from build123d import *

# Parameters (mm, degrees)
ESQUISSE1_R             = 50
ESQUISSE1_R_2           = 4.25
BOSS_EXTRU_1_DEPTH      = 3
ESQUISSE2_R             = 4.25
BOSS_EXTRU_2_DEPTH      = 25
ENL_V_MAT_EXTRU_1_DEPTH = 20
CONG_1_R                = 2


with BuildPart() as part:
    # Esquisse1 → Boss.-Extru.1 (new body)
    with BuildSketch(Plane(origin=(0, 0, 0), x_dir=(1, 0, 0), z_dir=(0, 1, 0))):
        with Locations(Location((0, 0, 0), (0, 0, 270))):
            Circle(ESQUISSE1_R)
        with Locations(Location((0, 0, 0), (0, 0, 270))):
            Circle(ESQUISSE1_R_2, mode=Mode.SUBTRACT)
    extrude(amount=BOSS_EXTRU_1_DEPTH)

    # Esquisse2 → Boss.-Extru.2 (add)
    with BuildSketch(Plane(origin=(0, 3, 0), x_dir=(1, 0, 0), z_dir=(0, 1, 0))):
        with BuildLine():
            Line((9.886859967, 1.5), (47.476309882, 1.5))
            ThreePointArc((47.476309882, 1.5), (47.5, 0), (47.476309882, -1.5))
            Line((47.476309882, -1.5), (9.886859967, -1.5))
            ThreePointArc((9.886859967, -1.5), (7.071067812, -7.071067812), (1.5, -9.886859967))
            Line((1.5, -9.886859967), (1.5, -47.476309882))
            ThreePointArc((1.5, -47.476309882), (0, -47.5), (-1.5, -47.476309882))
            Line((-1.5, -47.476309882), (-1.5, -9.886859967))
            ThreePointArc((-1.5, -9.886859967), (-7.071067812, -7.071067812), (-9.886859967, -1.5))
            Line((-9.886859967, -1.5), (-47.476309882, -1.5))
            ThreePointArc((-47.476309882, -1.5), (-47.5, 0), (-47.476309882, 1.5))
            Line((-47.476309882, 1.5), (-9.886859967, 1.5))
            ThreePointArc((-9.886859967, 1.5), (-7.071067812, 7.071067812), (-1.5, 9.886859967))
            Line((-1.5, 9.886859967), (-1.5, 47.476309882))
            ThreePointArc((-1.5, 47.476309882), (0, 47.5), (1.5, 47.476309882))
            Line((1.5, 47.476309882), (1.5, 9.886859967))
            ThreePointArc((1.5, 9.886859967), (7.071067812, 7.071067812), (9.886859967, 1.5))
        make_face()
        with Locations(Location((0, 0, 0), (0, 0, 270))):
            Circle(ESQUISSE2_R, mode=Mode.SUBTRACT)
    extrude(amount=BOSS_EXTRU_2_DEPTH)

    # Esquisse3 → Enlèv. mat.-Extru.1 (cut)
    with BuildSketch(Plane(origin=(0, 28, 0), x_dir=(1, 0, 0), z_dir=(0, 1, 0))):
        Polygon((7.736493607, 0), (3.868246804, 6.7), (-3.868246804, 6.7), (-7.736493607, 0), (-3.868246804, -6.7), (3.868246804, -6.7), align=None)
    extrude(amount=-ENL_V_MAT_EXTRU_1_DEPTH, mode=Mode.SUBTRACT)

    # Congé1
    cong_1_edges = [part.edges().sort_by_distance(p)[0] for p in [
        (0, 0, -50),
        (0, 0, -4.25),
    ]]
    fillet(cong_1_edges, radius=CONG_1_R)


solid = part.part
Verification items for the finished model (mm, model axes). A direction names the side the tool comes from. Coordinates: 2 decimals unless noted, no trailing zeros. Order: outer loops, then holes, each group sorted by start corner. A loop starts at its lowest first (then second) coordinate and runs counter-clockwise, first axis right, second up. Notation, with made-up numbers: (30, 80) -> (76, 80) arc R6 ccw to (76, 86) -> close; hole circle Ø1 at (-33.5, -36). An arc over 180 degrees is marked (long way). Put each result on its own line as item: value. Start each with the question number.
1. Cross-section at B-B, the plane y = 5.5. Record the boundary of the cut face in (x, z).
2. Material ranges on L1, parallel to X at y = 5.65, z = 0; L2, parallel to X at y = 26, z = 0, recorded low to high. Write a range as [from, to].
3. Cross-section at C-C, the plane y = 14. Record the boundary of the cut face in (x, z).
4. Cross-section at A-A, the plane x = 0. Record the boundary of the cut face in (y, z), then the cut area to 3 significant figures.
5. Go/stop test with flat-tipped pins: pin 1 Ø6 at (x, z) = (14.5, -24.5) entering from +Y; pin 2 Ø1.5 at (x, z) = (-18.5, 14) entering from -Y; pin 3 Ø5 at (x, y) = (-32.5, 22) entering from +Z; pin 4 Ø1 at (y, z) = (20, -8.5) entering from +X. Record where each tip stops, or that it passes through.
6. Access from +Z, -Z, +X, -X, +Y, -Y to the whole of each face (thin tool, end or side, straight path). Record for faces 5 (the flat face through (-10, 3, 10)), 6 (the flat face through (28, 15, -1.5)), 7 (the flat face through (-1.5, 15, -28)).
7. Mould release check, pull along X, two halves, no side actions. Record for faces 1 (the flat face through (-5.83, 18.14, 3.3)), 2 (the cylindrical face through (7.01, 15.32, -7.13)), 3 (the flat face through (1, 0, 10)), 4 (the flat face through (3.33, 8, 2.88)): released by +X, released by -X, zero draft, split by the parting line, or undercut.
Computed:
1. outline: (-47.48, -1.5) -> (-9.89, -1.5) arc R10 ccw to (-1.5, -9.89) -> (-1.5, -47.48) arc R47.5 ccw to (1.5, -47.48) -> (1.5, -9.89) arc R10 ccw to (9.89, -1.5) -> (47.48, -1.5) arc R47.5 ccw to (47.48, 1.5) -> (9.89, 1.5) arc R10 ccw to (1.5, 9.89) -> (1.5, 47.48) arc R47.5 ccw to (-1.5, 47.48) -> (-1.5, 9.89) arc R10 ccw to (-9.89, 1.5) -> (-47.48, 1.5) arc R47.5 ccw to start; hole circle Ø8.5 at (0, 0)
2. L1: [-47.5, -4.25], [4.25, 47.5]
2. L2: [-47.5, -7.74], [7.74, 47.5]
3. outline: (-47.48, -1.5) -> (-9.89, -1.5) arc R10 ccw to (-1.5, -9.89) -> (-1.5, -47.48) arc R47.5 ccw to (1.5, -47.48) -> (1.5, -9.89) arc R10 ccw to (9.89, -1.5) -> (47.48, -1.5) arc R47.5 ccw to (47.48, 1.5) -> (9.89, 1.5) arc R10 ccw to (1.5, 9.89) -> (1.5, 47.48) arc R47.5 ccw to (-1.5, 47.48) -> (-1.5, 9.89) arc R10 ccw to (-9.89, 1.5) -> (-47.48, 1.5) arc R47.5 ccw to start; hole (-7.74, 0) -> (-3.87, -6.7) -> (3.87, -6.7) -> (7.74, 0) -> (3.87, 6.7) -> (-3.87, 6.7) -> close
4. outline: (0, -48) arc R2 ccw to (2, -50) -> (3, -50) -> (3, -47.5) -> (28, -47.5) -> (28, -6.7) -> (8, -6.7) -> (8, -4.25) -> (2, -4.25) arc R2 ccw to (0, -6.25) -> close; (0, 6.25) arc R2 ccw to (2, 4.25) -> (8, 4.25) -> (8, 6.7) -> (28, 6.7) -> (28, 47.5) -> (3, 47.5) -> (3, 50) -> (2, 50) arc R2 ccw to (0, 48) -> close
4. area: 2,340 mm2
5. pin 1: y = 3
5. pin 2: y = 0
5. pin 3: z = 1.5
5. pin 4: x = 6
6. face 5: +Y
6. face 6: -Z, +X, +Y
6. face 7: -Z, -X, +Y
7. face 1: undercut
7. face 2: released by +X
7. face 3: zero draft
7. face 4: undercut
